```python
from build123d import *

# Parameters (mm, degrees)
SKETCH1_W               = 80
SKETCH1_H               = 12.7
BOSS_EXTRUDE1_DEPTH     = 6.35
SKETCH2_R               = 5.625
CUT_EXTRUDE1_DEPTH      = 7.35
CUT_EXTRUDE1_DEPTH_BACK = 7.35
SKETCH3_W               = 23.827822186
SKETCH3_H               = 5
CUT_EXTRUDE2_DEPTH      = 7.35
CUT_EXTRUDE2_DEPTH_BACK = 7.35
M4X0_7_TAPPED_HOLE1_D   = 3.3
GOO_DEPTH               = 0.5
BOSS_EXTRUDE5_DEPTH     = 1
F_3_0MM_DOWEL_HOLE1_D   = 3
M5X0_8_TAPPED_HOLE1_D   = 4.2


with BuildPart() as part:
    # Sketch1 → Boss-Extrude1 (new body, symmetric)
    with BuildSketch(Plane(origin=(0, 0, 0), x_dir=(0, 0, -1), z_dir=(1, 0, 0))):
        Rectangle(SKETCH1_W, SKETCH1_H)
    extrude(amount=BOSS_EXTRUDE1_DEPTH, both=True)

    # Sketch2 → Cut-Extrude1 (cut, two sides)
    with BuildSketch(Plane(origin=(0, 0, 0), x_dir=(0, 0, -1), z_dir=(1, 0, 0))) as cut_extrude1_sk:
        with Locations((-6.875, 0)):
            Circle(SKETCH2_R)
        with Locations((6.875, 0)):
            Circle(SKETCH2_R)
    extrude(amount=CUT_EXTRUDE1_DEPTH, mode=Mode.SUBTRACT)
    extrude(cut_extrude1_sk.sketch, amount=-CUT_EXTRUDE1_DEPTH_BACK, mode=Mode.SUBTRACT)

    # Sketch3 → Cut-Extrude2 (cut, two sides)
    with BuildSketch(Plane(origin=(0, 0, 0), x_dir=(0, 0, -1), z_dir=(1, 0, 0))) as cut_extrude2_sk:
        Rectangle(SKETCH3_W, SKETCH3_H)
    extrude(amount=CUT_EXTRUDE2_DEPTH, mode=Mode.SUBTRACT)
    extrude(cut_extrude2_sk.sketch, amount=-CUT_EXTRUDE2_DEPTH_BACK, mode=Mode.SUBTRACT)

    # M4x0.7 Tapped Hole1 (through all)
    with Locations(Plane(origin=(0, 6.35, 0), x_dir=(1, 0, 0), z_dir=(0, 1, 0))):
        with Locations((0, 35), (0, 20), (0, -20), (0, -35)):
            Hole(M4X0_7_TAPPED_HOLE1_D / 2)

    # Sketch8 → Goo (add, symmetric)
    with BuildSketch(Plane(origin=(0, 6.35, 0), x_dir=(1, 0, 0), z_dir=(0, 1, 0))):
        with BuildLine():
            Line((-5.13731221, -8.377770681), (-5.13731221, 8.377770681))
            ThreePointArc((-5.13731221, 8.377770681), (0, 13.515082891), (5.13731221, 8.377770681))
            Line((5.13731221, 8.377770681), (5.13731221, -8.377770681))
            ThreePointArc((5.13731221, -8.377770681), (0, -13.515082891), (-5.13731221, -8.377770681))
        make_face()
    goo = extrude(amount=GOO_DEPTH, both=True)

    # Mirror1: Goo across plane
    add(goo.mirror(Plane.ZX))

    # Sketch9 → Boss-Extrude5 (add, symmetric)
    with BuildSketch(Plane(origin=(6.35, 0, 0), x_dir=(0, 0, -1), z_dir=(1, 0, 0))):
        with BuildLine():
            Line((9.451941016, -5), (27.451941016, -5))
            Line((27.451941016, -5), (27.451941016, 5))
            Line((27.451941016, 5), (9.451941016, 5))
            ThreePointArc((9.451941016, 5), (12.5, 0), (9.451941016, -5))
        make_face()
    extrude(amount=BOSS_EXTRUDE5_DEPTH, both=True)

    # Ø3.0mm Dowel Hole1 (through all)
    with Locations(Plane.ZY.offset(6.35)):
        with Locations((-20, 0), (-35, 0)):
            Hole(F_3_0MM_DOWEL_HOLE1_D / 2)

    # M5x0.8 Tapped Hole1 (through all)
    with Locations(Plane(origin=(0, 6.35, 0), x_dir=(1, 0, 0), z_dir=(0, 1, 0))):
        with Locations((0, 35), (0, 20)):
            Hole(M5X0_8_TAPPED_HOLE1_D / 2)


solid = part.part
```
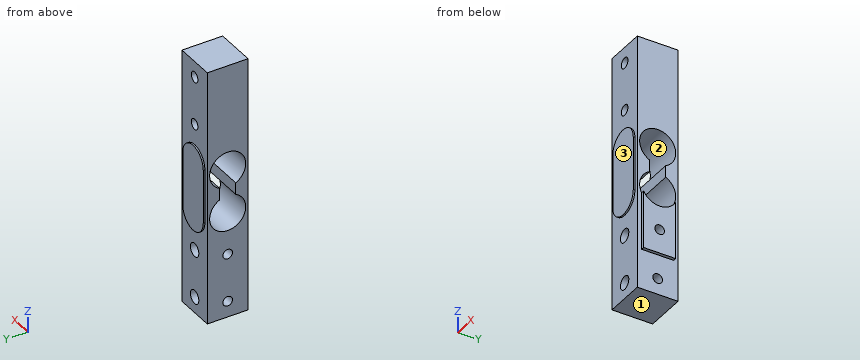
Geometry check sheet. Reference: the model listing, model coordinates, mm. Face numbers are marked on the shaded views. Coordinates: 2 decimals unless noted, no trailing zeros. Write each loop counter-clockwise with the first axis right and the second up, starting at its lowest first coordinate (ties: lowest second). Pieces come first, ordered by that corner, then holes. Notation, with made-up numbers: (45.5, -15) -> (60.5, -15) arc R19 cw to (60.5, 15) -> close; hole circle Ø5 at (57.5, 75). An arc over 180 degrees is marked (long way). Use CSV: the item, a comma, the result in double quotes. Start each with the question number.
Item 1: Cross-section at B-B, the plane y = 0. Record the cut outline in (x, z).
Item 2: Mould release check, pull along Z, two halves, no side actions. Record for the marked faces 1, 2 and 3: released by +Z, released by -Z, zero draft, split by the parting line, or undercut.
Item 3: Cross-section at C-C, the plane z = 35. Record the cut outline in (x, y), plus the area to 3 significant figures.
Item 4: Cross-section at A-A, the plane x = 0. State how many separate pieces and enclosed holes the cut face has, plus the area to 3 significant figures.
Item 5: Depth check by flat-ended pin: pin 1 Ø2.5 at (x, z) = (0, 20) entering from +Y; pin 2 Ø0.8 at (x, y) = (7, -0.5) entering from -Z; pin 3 Ø0.6 at (y, z) = (6.5, -1) entering from +X; pin 4 Ø3 at (x, z) = (-2, 25.5) entering from -Y. Enter the tip coordinate at first touch or a pass-through.
Item 6: Thickness scan on line 1 (Z direction, x = -3.5, y = 0); line 2 (Y direction, x = 3.5, z = -35); line 3 (Z direction, x = 0.25, y = 5.75). Record the ranges inside material, lowest first.
Item 7: Cross-section at D-D, the plane z = -35. Record the cut outline in (x, y), plus the area to 4 significant figures.
Answers:
1,outline,"(-6.35, -40) -> (6.35, -40) -> (6.35, -36.5) -> (1.47, -36.5) arc R2.1 cw to (-1.47, -36.5) -> (-6.35, -36.5) -> close; (-6.35, -33.5) -> (-1.47, -33.5) arc R2.1 cw to (1.47, -33.5) -> (6.35, -33.5) -> (6.35, -27.45) -> (7.35, -27.45) -> (7.35, -21.5) -> (1.47, -21.5) arc R2.1 cw to (-1.47, -21.5) -> (-6.35, -21.5) -> close; (-6.35, -18.5) -> (-1.47, -18.5) arc R2.1 cw to (1.47, -18.5) -> (7.35, -18.5) -> (7.35, -12.5) -> (-6.35, -12.5) -> close; (-6.35, 12.5) -> (6.35, 12.5) -> (6.35, 40) -> (-6.35, 40) -> close; hole circle Ø3.3 at (0, 20); hole circle Ø3.3 at (0, 35)"
2,face 1,"released by -Z"
2,face 2,"undercut"
2,face 3,"zero draft"
3,outline,"(-6.35, -6.35) -> (-1.65, -6.35) -> (-1.65, 6.35) -> (-6.35, 6.35) -> close; (1.65, -6.35) -> (6.35, -6.35) -> (6.35, 6.35) -> (1.65, 6.35) -> close"
3,area,"119 mm^2"
4,separate pieces,"5"
4,enclosed holes,"1"
4,area,"639 mm^2"
5,pin 1,"through"
5,pin 2,"z = -27.45"
5,pin 3,"x = 6.35"
5,pin 4,"y = -6.35"
6,line 1,"-40 to -36.5, -33.5 to -21.5, -18.5 to -12.5, 12.5 to 40"
6,line 2,"-6.35 to -1.5, 1.5 to 6.35"
6,line 3,"-40 to -37.09, -32.91 to -22.09, -17.91 to 18.37, 21.63 to 33.37, 36.63 to 40"
7,outline,"(-6.35, -6.35) -> (-2.1, -6.35) -> (-2.1, -1.5) -> (-6.35, -1.5) -> close; (-6.35, 1.5) -> (-2.1, 1.5) -> (-2.1, 6.35) -> (-6.35, 6.35) -> close; (2.1, -6.35) -> (6.35, -6.35) -> (6.35, -1.5) -> (2.1, -1.5) -> close; (2.1, 1.5) -> (6.35, 1.5) -> (6.35, 6.35) -> (2.1, 6.35) -> close"
7,area,"82.45 mm^2"
